Part model, mm, in its own coordinate system. A direction names the side the tool comes from. Round coordinates to 2 decimals unless told otherwise and drop trailing zeros. Write each loop counter-clockwise with the first axis right and the second up, starting at its lowest first coordinate (ties: lowest second). Pieces come first, ordered by that corner, then holes.
```python
from build123d import *

# Parameters (mm, degrees)
F0_W     = 22
F0_H     = 42
F0_W_2   = 20.2
F0_H_2   = 40.2
F1_DEPTH = 5
F2_W     = 20.2
F2_H     = 40.2
F3_DEPTH = 2
F4_R     = 0.8


with BuildPart() as f1:
    # F0 (on Top) → F1 (new body)
    with BuildSketch(Plane.XY):
        with Locations((11, 21)):
            Rectangle(F0_W, F0_H)
        with Locations((11, 21)):
            Rectangle(F0_W_2, F0_H_2, mode=Mode.SUBTRACT)
    extrude(amount=-F1_DEPTH)

    # F2 (on face) → F3 (join)
    with BuildSketch(Plane.XY):
        Polygon((0, 42), (0, 0), (22, 0), (22, 21), (22, 42), align=None)
        with Locations((11, 21)):
            Rectangle(F2_W, F2_H, mode=Mode.SUBTRACT)
        with Locations((11, 21)):
            Rectangle(F2_W, F2_H)
        with BuildLine():
            Line((22, 42), (22, 21))
            ThreePointArc((22, 21), (24.6191216351, 29.9495548074), (31.65, 36.075))
            Line((31.65, 36.075), (27.75, 42))
            Line((27.75, 42), (22, 42))
        make_face()
    extrude(amount=F3_DEPTH)

    # F4
    f4_edges = [f1.edges().sort_by_distance(p)[0] for p in [
        (22, 0, -1.5),
        (0, 0, -1.5),
        (0, 42, -1.5),
        (22, 42, -2.5),
        (21.1, 0.9, -2.5),
        (21.1, 41.1, -2.5),
        (0.9, 0.9, -2.5),
        (0.9, 41.1, -2.5),
    ]]
    fillet(f4_edges, radius=F4_R)


solid = f1.part
```
Q1. Mould opens along Y. For faces 4 (the cylindrical face through (21.77, 0.24, -1.45)), 5 (the cylindrical face through (20.86, 40.87, -2.54)), 6 (the flat face through (22, 21, -2)) say: +Y half, -Y half, draft (parallel to the pull), parting line (faces both ways), or undercut.
Values follow:
face 4: -Y half
face 5: undercut
face 6: draft
Q2. Cut at A-A on z = -1.5. Write the cut outline in (x, y).
Values follow:
outline: (0, 0.8) arc R0.8 ccw to (0.8, 0) - (21.2, 0) arc R0.8 ccw to (22, 0.8) - (22, 41.2) arc R0.8 ccw to (21.2, 42) - (0.8, 42) arc R0.8 ccw to (0, 41.2) - close; hole (0.9, 1.7) arc R0.8 ccw to (1.7, 0.9) - (20.3, 0.9) arc R0.8 ccw to (21.1, 1.7) - (21.1, 40.3) arc R0.8 ccw to (20.3, 41.1) - (1.7, 41.1) arc R0.8 ccw to (0.9, 40.3) - close
Q3. Wall check: L1, parallel to X at y = 10, z = -0.5; L2, parallel to Y at x = 5.5, z = -3.5; L3, parallel to X at y = 14, z = 1.5. Give the ranges that are in metal, low to high.
Values follow:
L1: x = 0 to 0.9, 21.1 to 22
L2: y = 0 to 0.9, 41.1 to 42
L3: x = 0 to 22
Q4. Which spindle directions (+Z, -Z, +X, -X, +Y, -Y) get a long thin tool onto all of the face, cutting with end or side? Do faces 1 (the flat face through (0, 21, -2)), 2 (the cylindrical face through (21.77, 41.76, -2.54)), 3 (the flat face through (0.9, 21, -2)). Say none if no direction does.
Values follow:
face 1: +Z, -Z, -X, +Y, -Y
face 2: -Z, +X, +Y
face 3: -Z
Q5. Drop a flat-ended pin along its axis: pin 1 (4 mm diameter, centred on x = 12, y = 34, fed in from -Z). Give the stop position or say it passes through.
Values follow:
pin 1: stops at z = 0
Q6. Cut at D-D on z = 0.5. Write the cut outline in (x, y) (3 decimals), plus the area to 3 significant figures.
Values follow:
outline: (0, 0.8) arc R0.8 ccw to (0.8, 0) - (21.2, 0) arc R0.8 ccw to (22, 0.8) - (22, 21) arc R16.6 cw to (31.65, 36.075) - (27.75, 42) - (0.8, 42) arc R0.8 ccw to (0, 41.2) - close
area: 1,010 mm2
Q7. Cut at C-C on x = 4. Write the cut outline in (y, z).
Values follow:
outline: (0, -5) - (0.9, -5) - (0.9, 0) - (41.1, 0) - (41.1, -5) - (42, -5) - (42, 2) - (0, 2) - close
Q8. Cut at B-B on y = 11. Write the cut outline in (x, z), plus the area to 3 significant figures.
Values follow:
outline: (0, -5) - (0.9, -5) - (0.9, 0) - (21.1, 0) - (21.1, -5) - (22, -5) - (22, 2) - (0, 2) - close
area: 53.0 mm2
